For this review, use the dimensioned drawing (mm, ordinates from the lowest corner) and the shaded views. A direction names the side the tool comes from. Coordinates: 2 decimals unless noted, no trailing zeros. Loops run counter-clockwise (first coordinate to the right, second up) from the corner with the lowest first, then second, coordinate; pieces in that order, holes last.
1. Mouldability with a two-part tool opening along X and no side actions: class the marked faces 1, 2, 3 and 4 as pulls with the +X half, pulls with the -X half, needs draft (parallel to the pull), parting line crosses it, or undercut.
2. Take a section at B-B, the plane y = 11.75. State the section outline as (x, z) points.
3. Machinability: for the marked faces 5, 6, 7, 8 and 9, which of the approach directions +Z, -Z, +X, -X, +Y, -Y give a long, thin tool a straight path to every point of the face, cutting with its end or side? Answer none if there is none.
4. Take a section at D-D, the plane x = 20. State the section outline as (y, z) points, then the cut area to 3 significant figures.
5. Clearance check with flat-ended pins moving along their axes: P1, Ø3, axis at y = 10.5, z = 25.5, coming from the -X side; P2, Ø5.5, axis at x = 29, z = 6, coming from the -Y side; P3, Ø3, axis at x = 30, z = 21, coming from the -Y side; P4, Ø3, axis at x = 5, z = 6, coming from the -Y side. State where each tip first meets the part, or that it passes through.
6. Take a section at A-A, the plane z = 6. State the section outline as (x, y) points.
7. To check wall thickness, follow probe 1 along Z at (x, y) = (29, 10.5); probe 2 along X at (y, z) = (16.25, 24); probe 3 along X at (y, z) = (9.5, 24). State the ranges of each line that lie inside material, in increasing order.
8. Take a section at C-C, the plane x = 29. State the section outline as (y, z) points.
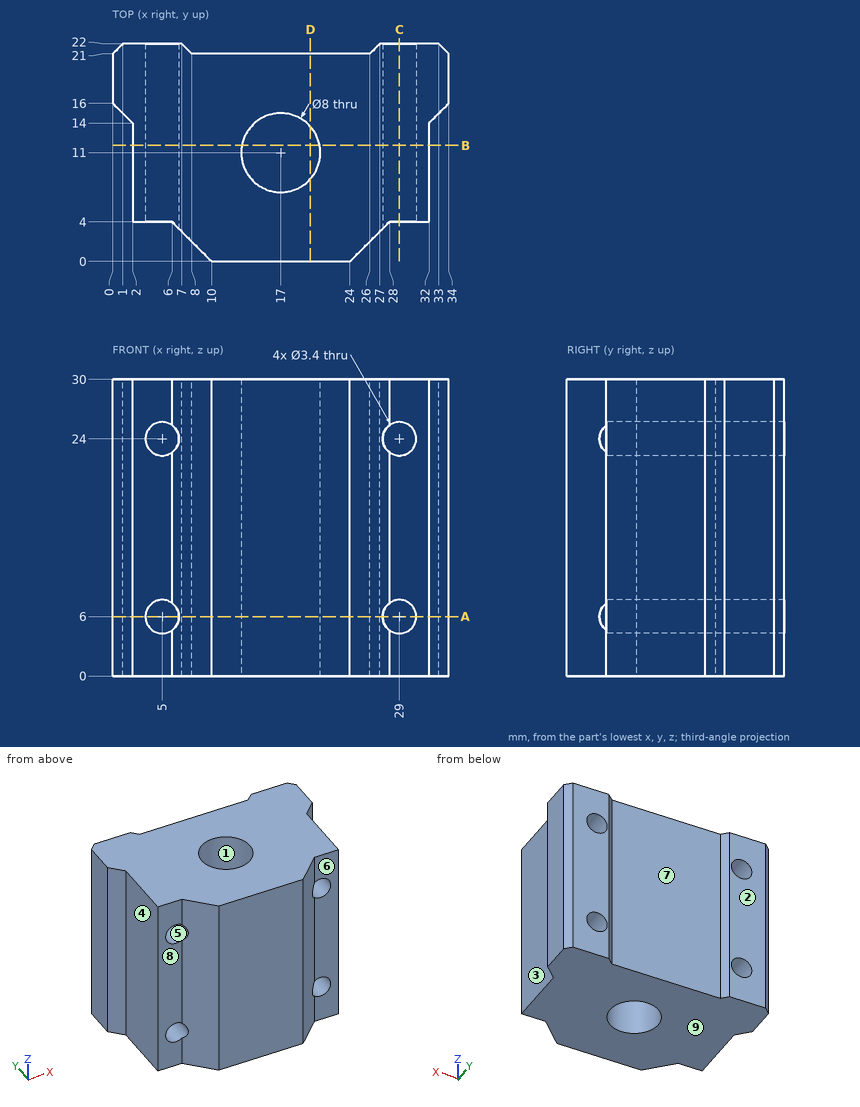
Results list:
1. face 1: undercut
1. face 2: needs draft
1. face 3: pulls with the +X half
1. face 4: pulls with the -X half
2. outline: (2, 0) - (13.07, 0) - (13.07, 30) - (2, 30) - close; (20.93, 0) - (32, 0) - (32, 30) - (20.93, 30) - close; hole circle Ø3.4 at (5, 6); hole circle Ø3.4 at (5, 24); hole circle Ø3.4 at (29, 6); hole circle Ø3.4 at (29, 24)
3. face 5: +Y, -Y
3. face 6: +Z, -Z, +X, -Y
3. face 7: +Z, -Z, +Y
3. face 8: +Z, -Z, -X, -Y
3. face 9: -Z, +X, -X, +Y, -Y
4. outline: (0, 0) - (8.35, 0) - (8.35, 30) - (0, 30) - close; (13.65, 0) - (21, 0) - (21, 30) - (13.65, 30) - close
4. area: 471 mm2
5. P1: stops at x = 2
5. P2: stops at y = 2.25
5. P3: stops at y = 4
5. P4: passes through
6. outline: (0, 16) - (2, 14) - (2, 4) - (3.3, 4) - (3.3, 22) - (1, 22) - (0, 21) - close; (6.7, 3.3) - (10, 0) - (24, 0) - (27.3, 3.3) - (27.3, 22) - (27, 22) - (26, 21) - (8, 21) - (7, 22) - (6.7, 22) - close; (30.7, 4) - (32, 4) - (32, 14) - (34, 16) - (34, 21) - (33, 22) - (30.7, 22) - close; hole circle Ø8 at (17, 11)
7. probe 1: z = 0 to 4.3, 7.7 to 22.3, 25.7 to 30
7. probe 2: x = 0 to 3.3, 6.7 to 27.3, 30.7 to 34
7. probe 3: x = 2 to 3.3, 6.7 to 13.29, 20.71 to 27.3, 30.7 to 32
8. outline: (4, 0) - (22, 0) - (22, 4.3) - (4, 4.3) - close; (4, 7.7) - (22, 7.7) - (22, 22.3) - (4, 22.3) - close; (4, 25.7) - (22, 25.7) - (22, 30) - (4, 30) - close
